Source: CAD feature listing. Evaluate the final solid. Frame: model axes, mm. Face numbers are marked on the shaded views. A direction names the side the tool comes from. Give positions to 0.01 mm unless a question says otherwise; leave off trailing zeros. Order: outer loops, then holes, each group sorted by start corner. A loop starts at its lowest first (then second) coordinate and runs counter-clockwise, first axis right, second up. Notation, with made-up numbers: M 0.5,80 L 17.5,80 A33 ccw 17.5,115 Z; hole C 1,51 d1. An arc over 180 degrees is marked long. Answer in a Markdown table with one row per item. Add a question column.
(1) Section query A-A, the plane x = 0. Return loops of the section in (y, z), plus the area to 3 significant figures.
(2) Material intervals for line 1 along Z through (x, y) = (0, 8.25); line 2 along X through (y, z) = (22.5, 0); line 3 along Z through (x, y) = (-2.75, 18), sorted ascending.
(3) Pin query (flat end, axial travel): P1, Ø2, axis at y = 3.5, z = 2, coming from the +X side; P2, Ø3.5, axis at y = 21.4, z = 0, coming from the +X side; P3, Ø6.5, axis at x = 0, z = 0, coming from the -Y side. Return the tip coordinate at first contact, or that it passes through.
(4) Section query C-C, the plane y = 22. Return loops of the section in (x, z), plus the area to 3 significant figures.
(5) Set-up query: the marked faces 5, 6 and 7. Return all of +Z, -Z, +X, -X, +Y, -Y with unobstructed straight access to the full face (end or side cutting, diameter ignored); none if empty.
(6) Section query B-B, the plane z = 0. Return loops of the section in (x, y).
(7) Mould query, pull axis Z, two halves, no side actions, for the marked faces 1, 2, 3 and 4. Classes: pulls with the +Z half, pulls with the -Z half, needs draft (parallel to the pull), parting line crosses it, or undercut.
(8) Section query D-D, the plane y = 12. Return loops of the section in (x, z), plus the area to 3 significant figures.
Autodesk Inventor part; units mm, degrees
ref_plane "Work Plane1" through (0, 0, 9.4) normal (0, 0, 1) x (1, 0, 0)
ref_plane "YZ Plane" through (0, 0, 0) normal (1, 0, 0) x (0, 1, 0)
ref_plane "XZ Plane" through (0, 0, 0) normal (0, 1, 0) x (-1, 0, 0)
sketch "Sketch1" plane through (0, 0, 0) normal (0, 1, 0) x (-1, 0, 0)
  circle A0 centre (0, 0) radius 9.4
  circle A1 centre (0, 0) radius 4
  circle A2 centre (0, 0) radius 2.5
  dimension "d0" = 8
  dimension "d1" = 18.8
  dimension "d2" = 5
extrude "Extrusion1" add sketch "Sketch1" along normal blind 25 contours A0 | A1
extrude "Extrusion2" cut sketch "Sketch1" along normal blind 18.5 contours A1
ref_plane "Work Plane1" through (0, 0, 9.4) normal (0, 0, 1) x (1, 0, 0)
sketch "Sketch2" plane through (0, 0, 9.4) normal (0, 0, 1) x (1, 0, 0)
  circle A0 centre (0, 21.4) radius 2
  circle A1 centre (0, 3.6) radius 2
  line L0 (9.4, 0) -> (-9.4, 0)
  line L1 (9.4, 25) -> (-9.4, 25)
  point P0 (0, 0)
  dimension "d7" = 4
  dimension "d8" = 3.6
  dimension "d9" = 3.6
extrude "Extrusion3" cut sketch "Sketch2" against normal up to next
pattern_circular "Circular Pattern1" count 2 over 90 about axis through (0, 0, 0) along (0, 1, 0) of "Extrusion3"
equation "\"d9\" = d8"
properties part number "Shaft coupler"
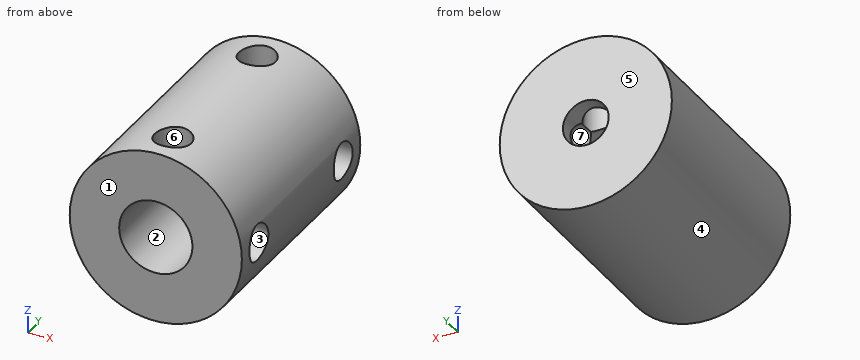
Values follow:
| question | item | result |
|---|---|---|
| 1 | outline | M 0,-9.4 L 25,-9.4 L 25,-2.5 L 18.5,-2.5 L 18.5,-4 L 0,-4 Z; M 0,4 L 1.6,4 L 1.6,9.4 L 0,9.4 Z; M 5.6,4 L 18.5,4 L 18.5,2.5 L 19.4,2.5 L 19.4,9.4 L 5.6,9.4 Z; M 23.4,2.5 L 25,2.5 L 25,9.4 L 23.4,9.4 Z |
| 1 | area | 240 mm² |
| 2 | line 1 | z = -9.4 to -4, 4 to 9.4 |
| 2 | line 2 | x = -9.4 to -2.5 |
| 2 | line 3 | z = -8.99 to -2.9, 2.9 to 8.99 |
| 3 | P1 | stops at x = 9.25 |
| 3 | P2 | stops at x = -1.79 |
| 3 | P3 | stops at y = 18.5 |
| 4 | outline | M -1.91,1.62 L -1.91,9.2 A9.4 ccw long 9.2,-1.91 L 1.62,-1.91 A2.5 cw Z; M 1.91,1.91 L 9.2,1.91 A9.4 ccw 1.91,9.2 Z |
| 4 | area | 204 mm² |
| 5 | face 5 | +Z, -Z, +X, -X, +Y |
| 5 | face 6 | +Z |
| 5 | face 7 | +X |
| 6 | outline | M -9.4,0 L -4,0 L -4,18.5 L -2.5,18.5 L -2.5,25 L -9.4,25 Z; M 2.5,18.5 L 4,18.5 L 4,5.6 L 9.4,5.6 L 9.4,19.4 L 2.5,19.4 Z; M 2.5,23.4 L 9.4,23.4 L 9.4,25 L 2.5,25 Z; M 4,0 L 9.4,0 L 9.4,1.6 L 4,1.6 Z |
| 7 | face 1 | needs draft |
| 7 | face 2 | undercut |
| 7 | face 3 | undercut |
| 7 | face 4 | parting line crosses it |
| 8 | outline | C 0,0 d18.8; hole C 0,0 d8 |
| 8 | area | 227 mm² |
